Autodesk Inventor part; units mm, degrees
ref_plane "YZ Plane" through (0, 0, 0) normal (1, 0, 0) x (0, 1, 0)
ref_plane "XZ Plane" through (0, 0, 0) normal (0, 1, 0) x (-1, 0, 0)
ref_plane "XY Plane" through (0, 0, 0) normal (0, 0, 1) x (1, 0, 0)
sketch "Sketch1" plane through (0, 0, 0) normal (0, 1, 0) x (-1, 0, 0)
  line L0 (0, -19.4583) -> (0, 19.4583) construction
  line L1 (5.5417, -19.4583) -> (5.5417, 19.4583) construction
  line L2 (-5.5417, 19.4583) -> (-5.5417, -19.4583) construction
  arc A0 (-5.5417, -19.4583) -> (5.5417, -19.4583) centre (0, -19.4583) ccw construction
  arc A1 (5.5417, 19.4583) -> (-5.5417, 19.4583) centre (0, 19.4583) ccw construction
  line L3 (-5.4417, 19.4583) -> (-5.4417, -19.4583)
  arc A2 (-5.4417, -19.4583) -> (5.4417, -19.4583) centre (0, -19.4583) ccw
  line L4 (5.4417, -19.4583) -> (5.4417, 19.4583)
  arc A3 (5.4417, 19.4583) -> (-5.4417, 19.4583) centre (0, 19.4583) ccw
  point P0 (0, 0)
  dimension "d0" = 5.5417
  dimension "d1" = 38.9167
  dimension "d2" = 0.1
extrude "Extrusion1" add sketch "Sketch1" along normal blind 48.3333
chamfer "Chamfer1" distance 3 angle 45 4 edges at (5.4417, 0, 0) (0, 0, -24.9) (-5.4417, 0, 0) (0, 0, 24.9)
fillet "Fillet2" radius 10.24 4 edges at (0, 3, 24.9) (-5.4417, 3, 0) (0, 3, -24.9) (5.4417, 3, 0)
properties part number "Contenedor anti-fuga (para imprimir en modo espiral)"
CAD build for the part. Positions are in the model's coordinates, mm. Round coordinates to 2 decimals unless told otherwise and drop trailing zeros. Order: outer loops, then holes, each group sorted by start corner. A loop starts at its lowest first (then second) coordinate and runs counter-clockwise, first axis right, second up. Notation, with made-up numbers: (61, -17.5) -> (78, -17.5) arc R31 cw to (78, 13.5) -> close; hole circle Ø7 at (69.25, 14). An arc over 180 degrees is marked (long way). Write item = value, one per line. Start each with the question number.
(1) Cut at B-B, the plane y = 14. List the corners of the cut face in (x, z).
(2) Pin check, flat tip, straight feed: P1, Ø8, axis at y = 5, z = 9, coming from the -X side. Stop position of the tip, or through.
(3) Probe line 1 (X direction, y = 7, z = -10.5); line 2 (X direction, y = 4.5, z = 11.5); line 3 (Z direction, x = -2.75, y = 5). List the from-to ranges inside material, lowest first. Write a range as [from, to].
Model answer:
q1.outline = (-5.44, -19.46) arc R5.44 ccw to (5.44, -19.46) -> (5.44, 19.46) arc R5.44 ccw to (-5.44, 19.46) -> close
q2.P1 = -5.44
q3.line_1 = [-5.44, 5.44]
q3.line_2 = [-5.07, 5.07]
q3.line_3 = [-23.86, 23.86]
